The model under review builds one solid part; all positions refer to its coordinate system, in mm. A direction names the side the tool comes from. Give positions to 0.01 mm unless a question says otherwise; leave off trailing zeros. Write each loop counter-clockwise with the first axis right and the second up, starting at its lowest first coordinate (ties: lowest second). Pieces come first, ordered by that corner, then holes. Notation, with made-up numbers: (37, 25.5) -> (45, 25.5) arc R11 cw to (45, 38.5) -> close; hole circle Ø5 at (-29, 9.25). An arc over 180 degrees is marked (long way). Use CSV: the item, a comma, the result in double quotes.
```python
from build123d import *

# Parameters (mm, degrees)
SKETCH1_W           = 30
SKETCH1_H           = 15.5
BOSS_EXTRUDE1_DEPTH = 1
SKETCH2_R           = 1
BOSS_EXTRUDE2_DEPTH = 9
SKETCH3_W           = 4.279397372
SKETCH3_H           = 3.040773008
BOSS_EXTRUDE3_DEPTH = 3


with BuildPart() as part:
    # Sketch1 → Boss-Extrude1 (new body)
    with BuildSketch(Plane(origin=(0, 0, 0), x_dir=(1, 0, 0), z_dir=(0, 1, 0))):
        with Locations((1.743407461, -3.928718986)):
            Rectangle(SKETCH1_W, SKETCH1_H)
    extrude(amount=BOSS_EXTRUDE1_DEPTH)

    # Sketch2 → Boss-Extrude2 (add)
    with BuildSketch(Plane.ZY.offset(13.256592539)):
        with Locations(Location((-0.717776519, 0.5, 0), (0, 0, 150))):
            Circle(SKETCH2_R)
        with Locations(Location((6.326509059, 0.5, 0), (0, 0, 150))):
            Circle(SKETCH2_R)
    extrude(amount=BOSS_EXTRUDE2_DEPTH)

    # Sketch3 → Boss-Extrude3 (add)
    with BuildSketch(Plane(origin=(0, 1, 0), x_dir=(1, 0, 0), z_dir=(0, 1, 0))):
        with Locations((2.821431472, 1.520386504)):
            Rectangle(SKETCH3_W, SKETCH3_H)
    extrude(amount=BOSS_EXTRUDE3_DEPTH)


solid = part.part
```
Q1. Consider section D-D (y = 3.6). Write out the cut boundary in (x, z).
Derived:
outline,"(0.68, -3.04) -> (4.96, -3.04) -> (4.96, 0) -> (0.68, 0) -> close"
Q2. Consider section B-B (z = -0.75). Write out the cut boundary in (x, y), then the cut area to 3 significant figures.
Derived:
outline,"(-22.26, -0.5) -> (-13.26, -0.5) -> (-13.26, 0) -> (16.74, 0) -> (16.74, 1) -> (4.96, 1) -> (4.96, 4) -> (0.68, 4) -> (0.68, 1) -> (-13.26, 1) -> (-13.26, 1.5) -> (-22.26, 1.5) -> close"
area,"60.8 mm2"
Q3. To check wall thickness, follow probe 1 along Y at (x, z) = (-6, 0.5); probe 2 along Y at (x, z) = (3, -3); probe 3 along X at (y, z) = (1.7, -1.5). State the ranges of each line that lie inside material, in increasing order.
Derived:
probe 1,"y = 0 to 1"
probe 2,"y = 0 to 4"
probe 3,"x = 0.68 to 4.96"
Q4. Insertion check: pin 1 (1.1 mm diameter, centred on y = 0.5, z = 3.5, fed in from -X); pin 2 (4.5 mm diameter, centred on x = 1, z = 6, fed in from -Y); pin 3 (1.5 mm diameter, centred on x = 2, y = 2, fed in from -Z); pin 4 (2 mm diameter, centred on x = -18, z = 0, fed in from -Y). Each pin has a flat end and moves straight along its axis. Give the tip position at first contact, or say it passes through.
Derived:
pin 1,"stops at x = -13.26"
pin 2,"stops at y = 0"
pin 3,"stops at z = -3.04"
pin 4,"stops at y = -0.5"
Q5. The part is to be moulded in two halves that separate along Z. For faces 1 (the flat face through (3, 2, -3.041)), 2 (the flat face through (3, 2, 0)), 3 (the flat face through (-13.257, 0.5, 2.8)), 4 (the flat face through (-13.257, 0.5, -2.7)), say which applies: pulls with the +Z half, pulls with the -Z half, needs draft (parallel to the pull), parting line crosses it, or undercut.
Derived:
face 1,"pulls with the -Z half"
face 2,"pulls with the +Z half"
face 3,"undercut"
face 4,"needs draft"
Q6. Machinability: for faces 5 (the cylindrical face through (-17.69, 1.5, 6.37)), 6 (the flat face through (4.961, 2, -1)), 7 (the flat face through (2, 0, 4)), 8 (the flat face through (-22.257, 0, -1)), which of the approach directions +Z, -Z, +X, -X, +Y, -Y give a long, thin tool a straight path to every point of the face, cutting with its end or side? Answer none if there is none.
Derived:
face 5,"-X"
face 6,"+Z, -Z, +X, +Y"
face 7,"+Z, -Z, +X, -Y"
face 8,"+Z, -Z, -X, +Y, -Y"
Q7. Consider section C-C (x = 13.5). Write out the cut boundary in (y, z).
Derived:
outline,"(0, -3.82) -> (1, -3.82) -> (1, 11.68) -> (0, 11.68) -> close"
Q8. Consider section A-A (y = 0.5). Write out the cut boundary in (x, z), then the cut area to 3 significant figures.
Derived:
outline,"(-22.26, -1.72) -> (-13.26, -1.72) -> (-13.26, -3.82) -> (16.74, -3.82) -> (16.74, 11.68) -> (-13.26, 11.68) -> (-13.26, 7.33) -> (-22.26, 7.33) -> (-22.26, 5.33) -> (-13.26, 5.33) -> (-13.26, 0.28) -> (-22.26, 0.28) -> close"
area,"501 mm2"
